The drawing under review shows one solid part. Ordinate dimensions are in mm from its lowest x, y, z. A direction names the side the tool comes from. Coordinates: 2 decimals unless noted, no trailing zeros. Write each loop counter-clockwise with the first axis right and the second up, starting at its lowest first coordinate (ties: lowest second). Pieces come first, ordered by that corner, then holes. Notation, with made-up numbers: (-21.75, -35.75) - (-14.75, -35.75) arc R16 cw to (-14.75, -25.75) - close; hole circle Ø9 at (13.25, -22.75). An arc over 180 degrees is marked (long way). Answer as CSV lines item,"result". Start each with the question number.
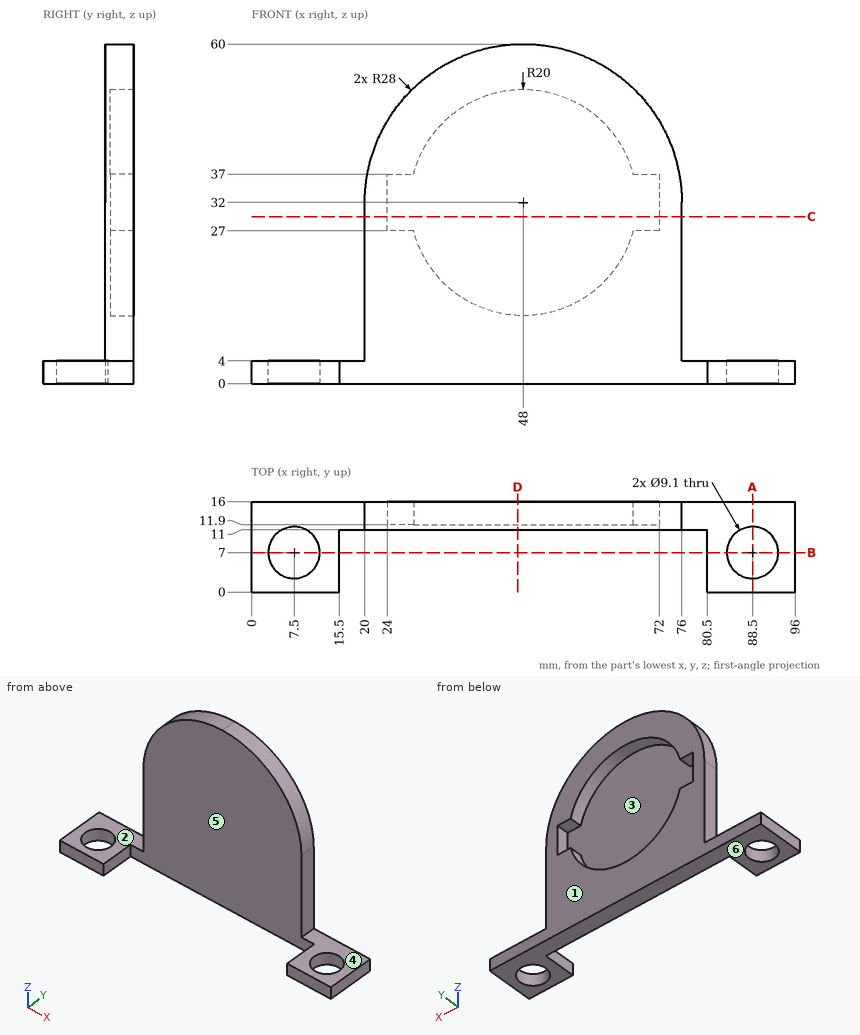
(1) Add section D-D on x = 47. Give the boundary of the cut face in (y, z) (3 decimals).
(2) For the marked faces 1 and 2, list the 3-axis set-ups (+Z, -Z, +X, -X, +Y, -Y) from which the entire face can be reached by the end or side of a thin tool; tool diameter is ignored.
(3) Wall thickness on line 1 (Y direction, x = 88.5, z = 2.6); line 2 (Y direction, x = 57, z = 10.5); line 3 (Z direction, x = 14.5, y = 7.75): over which ranges is each line inside the solid? List them lowest first.
(4) Add section C-C on z = 29.5. Give the boundary of the cut face in (x, y), then the cut area to 3 significant figures.
(5) The part is to be moulded in two halves that separate along Z. For the marked faces 3, 4, 5 and 6, say which applies: released by +Z, released by -Z, zero draft, split by the parting line, or undercut.
(6) For pin 1 (1.2 mm diameter, centred on y = 13.5, z = 33.5, fed in from -X); pin 2 (12 mm diameter, centred on x = 17.5, z = 31.5, fed in from -Y); pin 3 (5 mm diameter, centred on x = 81.5, y = 5.5, fed in from +Z); pin 4 (3.5 mm diameter, centred on x = 71, y = 14, fed in from -Z), all flat-tipped, find the tip position at first contact; note any pin that passes through.
(7) Add section B-B on y = 7. Give the boundary of the cut face in (x, z).
(8) Add section A-A on x = 88.5. Give the boundary of the cut face in (y, z), then the cut area to 3 significant figures.
Reported:
1,outline,"(11, 0) - (16, 0) - (16, 12.025) - (11.9, 12.025) - (11.9, 51.975) - (16, 51.975) - (16, 59.982) - (11, 59.982) - close"
2,face 1,"+Z, -Z, +X, -X, +Y"
2,face 2,"+Z, -X, +Y, -Y"
3,line 1,"0 to 2.45, 11.55 to 16"
3,line 2,"11 to 16"
3,line 3,"0 to 4"
4,outline,"(20, 11) - (76, 11) - (76, 16) - (72, 16) - (72, 11.9) - (24, 11.9) - (24, 16) - (20, 16) - close"
4,area,"83.2 mm²"
5,face 3,"undercut"
5,face 4,"released by +Z"
5,face 5,"zero draft"
5,face 6,"released by -Z"
6,pin 1,"x = 20.01"
6,pin 2,"y = 11"
6,pin 3,"z = 4"
6,pin 4,"z = 0"
7,outline,"(0, 0) - (2.95, 0) - (2.95, 4) - (0, 4) - close; (12.05, 0) - (15.5, 0) - (15.5, 4) - (12.05, 4) - close; (80.5, 0) - (83.95, 0) - (83.95, 4) - (80.5, 4) - close; (93.05, 0) - (96, 0) - (96, 4) - (93.05, 4) - close"
8,outline,"(0, 0) - (2.45, 0) - (2.45, 4) - (0, 4) - close; (11.55, 0) - (16, 0) - (16, 4) - (11.55, 4) - close"
8,area,"27.6 mm²"
